Model file for the job. Use its own axes, mm. Face numbers are marked on the shaded views. A direction names the side the tool comes from. Round coordinates to 2 decimals unless told otherwise and drop trailing zeros. Write each loop counter-clockwise with the first axis right and the second up, starting at its lowest first coordinate (ties: lowest second). Pieces come first, ordered by that corner, then holes. Notation, with made-up numbers: (3.25, 37.5) - (36.25, 37.5) arc R19 cw to (36.25, 71.5) - close; hole circle Ø4 at (45, 79.5). An arc over 180 degrees is marked (long way). Answer as a JSON object with one key per item and string values. Group by question number.
from build123d import *

# Parameters (mm, degrees)
SKETCH_W        = 70
SKETCH_H        = 30
SKETCH_R        = 1.75
SKETCH_W_2      = 15
SKETCH_H_2      = 20
PAD_DEPTH       = 6
FILLET_R        = 10
FILLET001_R     = 1
SKETCH001_W     = 5
SKETCH001_H     = 30
PAD001_DEPTH    = 40
CHAMFER_SIZE2   = 38
CHAMFER_SIZE    = 10
SKETCH002_R     = 2
POCKET_DEPTH    = 4
CHAMFER001_SIZE = 0.5
FILLET002_R     = 10
FILLET003_R     = 2
FILLET004_R     = 6
SKETCH003_R     = 2
POCKET001_DEPTH = 70.001
SKETCH004_R     = 2.25
POCKET002_DEPTH = 4
CHAMFER002_SIZE = 0.5


with BuildPart() as part:
    # Sketch → Pad (new body)
    with BuildSketch(Plane.XY):
        with Locations((25, 0)):
            Rectangle(SKETCH_W, SKETCH_H)
        Circle(SKETCH_R, mode=Mode.SUBTRACT)
        with Locations((40, 0)):
            Circle(SKETCH_R, mode=Mode.SUBTRACT)
        with Locations((20, 0)):
            Rectangle(SKETCH_W_2, SKETCH_H_2, mode=Mode.SUBTRACT)
    extrude(amount=PAD_DEPTH)

    # Fillet
    fillet_edges = [part.edges().sort_by_distance(p)[0] for p in [
        (-10, 15, 3),
        (-10, -15, 3),
    ]]
    fillet(fillet_edges, radius=FILLET_R)

    # Fillet001
    fillet001_edges = [part.edges().sort_by_distance(p)[0] for p in [
        (12.5, 0, 6),
        (12.5, 0, 0),
        (20, 10, 0),
        (20, 10, 6),
        (27.5, 0, 6),
        (20, -10, 6),
        (27.5, 0, 0),
        (20, -10, 0),
    ]]
    fillet(fillet001_edges, radius=FILLET001_R)

    # Sketch001 (on Face18 of Fillet001) → Pad001 (join)
    with BuildSketch(Plane.XY.offset(6)):
        with Locations((57.5, 0)):
            Rectangle(SKETCH001_W, SKETCH001_H)
    extrude(amount=PAD001_DEPTH)

    # Chamfer
    chamfer_edges = [part.edges().sort_by_distance(p)[0] for p in [
        (57.5, -15, 46),
        (57.5, 15, 46),
    ]]
    chamfer_side = part.faces().sort_by_distance((57.5, 0, 46))[0]
    chamfer(chamfer_edges, length=CHAMFER_SIZE, length2=CHAMFER_SIZE2, reference=chamfer_side)

    # Sketch002 (on Face4 of Chamfer) → Pocket (cut)
    with BuildSketch(Plane.XY.offset(6)):
        Circle(SKETCH002_R)
        with Locations((40, 0)):
            Circle(SKETCH002_R)
    extrude(amount=-POCKET_DEPTH, mode=Mode.SUBTRACT)

    # Chamfer001
    chamfer001_edges = [part.edges().sort_by_distance(p)[0] for p in [
        (-2, 0, 6),
        (38, 0, 6),
    ]]
    chamfer(chamfer001_edges, length=CHAMFER001_SIZE)

    # Fillet002
    fillet002_edges = [part.edges().sort_by_distance(p)[0] for p in [
        (55, 0, 6),
    ]]
    fillet(fillet002_edges, radius=FILLET002_R)

    # Fillet003
    fillet003_edges = [part.edges().sort_by_distance(p)[0] for p in [
        (60, 0, 0),
    ]]
    fillet(fillet003_edges, radius=FILLET003_R)

    # Fillet004
    fillet004_edges = [part.edges().sort_by_distance(p)[0] for p in [
        (57.5, -5, 46),
        (57.5, 5, 46),
    ]]
    fillet(fillet004_edges, radius=FILLET004_R)

    # Sketch003 (on Face2 of Fillet003) → Pocket001 (cut, through all)
    with BuildSketch(Plane.YZ.offset(60)):
        with Locations((0, 40)):
            Circle(SKETCH003_R)
        with Locations((0, 25)):
            Circle(SKETCH003_R)
    extrude(amount=-POCKET001_DEPTH, mode=Mode.SUBTRACT)

    # Sketch004 (on Face12 of Pocket001) → Pocket002 (cut)
    with BuildSketch(Plane(origin=(55, 0, 0), x_dir=(0, -1, 0), z_dir=(-1, 0, 0))):
        with Locations((0, 40)):
            Circle(SKETCH004_R)
        with Locations((0, 25)):
            Circle(SKETCH004_R)
    extrude(amount=-POCKET002_DEPTH, mode=Mode.SUBTRACT)

    # Chamfer002
    chamfer002_edges = [part.edges().sort_by_distance(p)[0] for p in [
        (55, 2.25, 40),
        (55, 2.25, 25),
    ]]
    chamfer(chamfer002_edges, length=CHAMFER002_SIZE)


solid = part.part
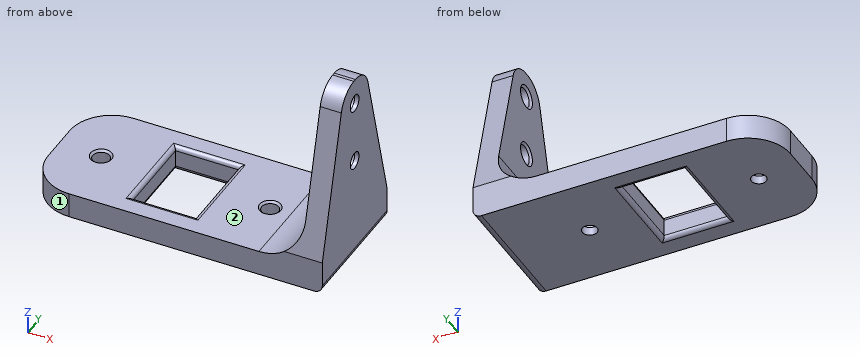
(1) Slice it at C-C (y = -7). Write the cut outline in (x, z).
(2) Slice it at A-A (x = 25). Write the cut outline in (y, z), then the cut area to 3 significant figures.
(3) Flat gauge pins, fed straight in: pin 1 (5 mm diameter, centred on x = 2, y = 11, fed in from +Z); pin 2 (6 mm diameter, centred on y = 0, z = 25, fed in from -X); pin 3 (2 mm diameter, centred on x = 45.5, y = -11.5, fed in from +Z). Where does each tip first touch, or does it go through?
(4) Slice it at D-D (x = 40). Write the cut outline in (y, z).
(5) Slice it at B-B (z = 25). Write the cut outline in (x, y), then the cut area to 3 significant figures.
(6) 3-axis set-ups, long thin cutter, end or side, ignore diameter. For the marked faces 1 and 2: which of +Z, -Z, +X, -X, +Y, -Y reach the whole face in a straight line?
(7) Drill centre lines: line 1 (Z direction, x = 56.35, y = 0); line 2 (Y direction, x = 40, z = 4); line 3 (Y direction, x = 20.5, z = 2.5). Where is each one in solid material? Low to high. Write a range as from..to.
Answer:
{
 "1": {"outline": "(-9.8, 0) - (11.5, 0) arc R1 ccw to (12.5, 1) - (12.5, 5) arc R1 ccw to (11.5, 6) - (-9.8, 6) - close; (27.5, 1) arc R1 ccw to (28.5, 0) - (58, 0) arc R2 ccw to (60, 2) - (60, 38.4) - (55, 38.4) - (55, 16) arc R10 cw to (45, 6) - (28.5, 6) arc R1 ccw to (27.5, 5) - close"},
 "2": {"outline": "(-15, 0) - (-11, 0) arc R1 ccw to (-10, 1) - (-10, 5) arc R1 ccw to (-11, 6) - (-15, 6) - close; (10, 1) arc R1 ccw to (11, 0) - (15, 0) - (15, 6) - (11, 6) arc R1 ccw to (10, 5) - close", "area": "59.1 mm²"},
 "3": {"pin 1": "z = 6", "pin 2": "x = 55", "pin 3": "z = 6.11"},
 "4": {"outline": "(-15, 0) - (-1.75, 0) - (-1.75, 2) - (-2, 2) - (-2, 5.5) - (-2.5, 6) - (-15, 6) - close; (1.75, 0) - (15, 0) - (15, 6) - (2.5, 6) - (2, 5.5) - (2, 2) - (1.75, 2) - close"},
 "5": {"outline": "(55, -10.53) - (60, -10.53) - (60, -2) - (59, -2) - (59, -2.25) - (55.5, -2.25) - (55, -2.75) - close; (55, 2.75) - (55.5, 2.25) - (59, 2.25) - (59, 2) - (60, 2) - (60, 10.53) - (55, 10.53) - close", "area": "83.0 mm²"},
 "6": {"face 1": "+Z, -Z, -X, -Y", "face 2": "+Z, -X, +Y, -Y"},
 "7": {"line 1": "0..22.75, 27.25..37.75, 42.25..46", "line 2": "-15..-2, 2..15", "line 3": "-15..-10, 10..15"}
}
